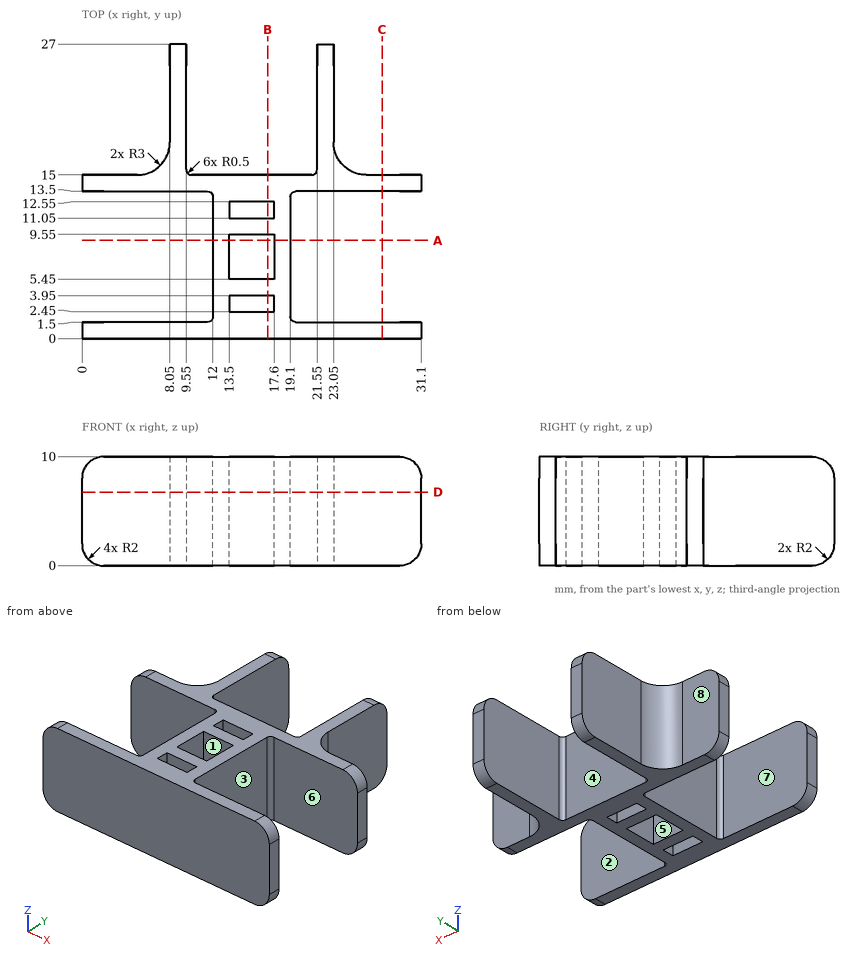
Input: dimensioned drawing with shaded views. Units: mm. Origin: part minimum x, y, z. A direction names the side the tool comes from. Give positions to 0.01 mm unless a question says otherwise; leave off trailing zeros. Order: outer loops, then holes, each group sorted by start corner. A loop starts at its lowest first (then second) coordinate and runs counter-clockwise, first axis right, second up. Notation, with made-up numbers: (88, 41.5) -> (103, 41.5) arc R21 cw to (103, 59.5) -> close; hole circle Ø8 at (43, -8.75). An arc over 180 degrees is marked (long way). Use a Markdown table: item, result.
1) Section query B-B, the plane x = 17. Return the cut outline in (y, z), then the cut area to 3 significant figures.
Answer list:
| item | result |
|---|---|
| outline | (0, 0) -> (2.45, 0) -> (2.45, 10) -> (0, 10) -> close; (3.95, 0) -> (5.45, 0) -> (5.45, 10) -> (3.95, 10) -> close; (9.55, 0) -> (11.05, 0) -> (11.05, 10) -> (9.55, 10) -> close; (12.55, 0) -> (15, 0) -> (15, 10) -> (12.55, 10) -> close |
| area | 79.0 mm² |
2) Section query C-C, the plane x = 27.5. Return the cut outline in (y, z), then the cut area to 3 significant figures.
Answer list:
| item | result |
|---|---|
| outline | (0, 0) -> (1.5, 0) -> (1.5, 10) -> (0, 10) -> close; (13.5, 0) -> (15, 0) -> (15, 10) -> (13.5, 10) -> close |
| area | 30.0 mm² |
3) Mould query, pull axis X, two halves, no side actions, for the marked faces 1, 2 and 3. Classes: +X half, -X half, draft (parallel to the pull), parting line (faces both ways), or undercut.
Answer list:
| item | result |
|---|---|
| face 1 | undercut |
| face 2 | draft |
| face 3 | +X half |
4) Section query D-D, the plane z = 6.75. Count the separate pieces of the cut face and the enclosed holes in it, then the cut area to 3 significant figures.
Answer list:
| item | result |
|---|---|
| separate pieces | 1 |
| enclosed holes | 3 |
| area | 190 mm² |
5) Contact query for flat-ended pins moving along their axis: P1, Ø3, axis at y = 6, z = 7, coming from the -X side; P2, Ø6, axis at x = 27, z = 4, coming from the +Y side; P3, Ø3.5, axis at x = 16.5, z = 6.5, coming from the +Y side. Output: stop coordinate, or through.
Answer list:
| item | result |
|---|---|
| P1 | x = 12 |
| P2 | y = 15.81 |
| P3 | y = 15 |
6) Ray query, line 1 along Y through (x, z) = (16.5, 9.5); line 2 along Y through (x, z) = (3, 5.5); line 3 along X through (y, z) = (19, 5.75). Return the intervals inside material, ascending. Write a range as [from, to].
Answer list:
| item | result |
|---|---|
| line 1 | [0, 2.45], [3.95, 5.45], [9.55, 11.05], [12.55, 15] |
| line 2 | [0, 1.5], [13.5, 15] |
| line 3 | [8.05, 9.55], [21.55, 23.05] |
7) Reachability of the marked faces 4, 5, 6, 7 and 8 from +Z, -Z, +X, -X, +Y, -Y: full face, straight path, thin tool, end or side. Return the list, or none.
Answer list:
| item | result |
|---|---|
| face 4 | +Z, -Z, +Y |
| face 5 | +Z, -Z |
| face 6 | +Z, -Z, +X |
| face 7 | +Z, -Z, -X |
| face 8 | +Z, -Z, -X, +Y |
8) Section query A-A, the plane y = 9. Return the cut outline in (x, z).
Answer list:
| item | result |
|---|---|
| outline | (12, 0) -> (13.5, 0) -> (13.5, 10) -> (12, 10) -> close; (17.6, 0) -> (19.1, 0) -> (19.1, 10) -> (17.6, 10) -> close |
